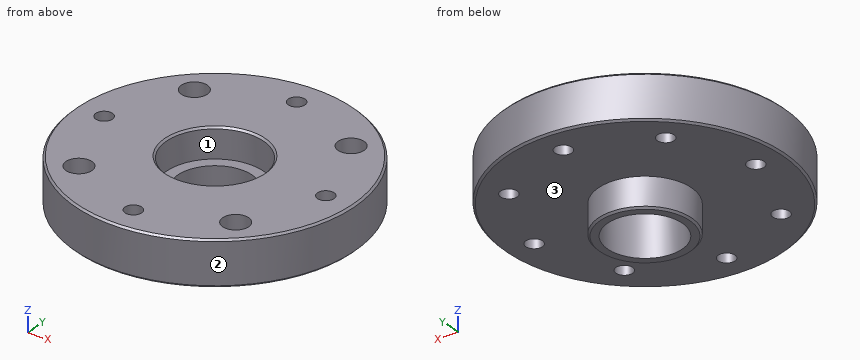
Solid Edge part; units mm, degrees
sketch "Sketch1" plane through (60.3162, 60.3162, 0) normal (0, 0, 1) x (1, 0, 0)
  circle A0 centre (-60.3162, -60.3162) radius 37.5
  circle A1 centre (-60.3162, -60.3162) radius 10
extrude "Protrusion1" add sketch "Sketch1" along normal blind 12
sketch "Sketch2" plane through (0, 0, 0) normal (0, 0, -1) x (1, 0, 0)
  circle A0 centre (0, 0) radius 10
  circle A1 centre (0, 0) radius 12.5
extrude "Extrusionsausprägung_2" add sketch "Sketch2" along normal blind 8
chamfer "Fase_1" distance 0.5 angle 45 1 edges at (-12.5, 0, -8)
hole "Bohrung_1" at (-30, 0, 12) direction (0, 0, -1) diameter 4.5 end through all
pattern_circular "Pattern1" count 8 over 360 about axis through (0, 0, 12) along (0, 0, 1) of "Bohrung_1"
chamfer "Fase_2" distance 0.5 angle 45 2 edges at (-37.5, 0, 12) (-37.5, 0, 0)
sketch "Sketch3" plane through (0, 0, 12) normal (0, 0, 1) x (-1, 0, 0)
  circle A0 centre (0, 0) radius 11
extrude "Extrusionsausprägung_4" add sketch "Sketch3" against normal blind 7
sketch "Sketch4" plane through (0, 0, 12) normal (0, 0, 1) x (-1, 0, 0)
  circle A0 centre (0, 0) radius 13
extrude "Extrusionsausschnitt_2" cut sketch "Sketch4" against normal blind 8
chamfer "Fase_3" distance 0.5 angle 45 1 edges at (13, 0, 12)
hole "Bohrung_2" at (-21.2132, -21.2132, 12) direction (0, 0, -1) diameter 4.5 end up to next counterbore diameter 7 counterbore depth 4
pattern_circular "Pattern3" count 4 over 360 about axis through (0, 0, 12) along (0, 0, -1) of "Bohrung_2"
properties material "Aluminium, 1060"
Design review of the part built by this model. Coordinates are the model's own, in mm. Face numbers are marked on the shaded views. A direction names the side the tool comes from. Round coordinates to 2 decimals unless told otherwise and drop trailing zeros. Order: outer loops, then holes, each group sorted by start corner. A loop starts at its lowest first (then second) coordinate and runs counter-clockwise, first axis right, second up. Notation, with made-up numbers: (56, 59.25) - (72, 59.25) arc R12 ccw to (72, 73.25) - close; hole circle Ø10 at (7, 36.5). An arc over 180 degrees is marked (long way). Return JSON: item names as keys, results as strings.
Q1. Consider section D-D on z = -5.75. Write out the cut boundary in (x, y).
Computed values:
{"outline": "circle Ø25 at (0, 0); hole circle Ø20 at (0, 0)"}
Q2. Wall thickness on L1, parallel to Y at x = 0, z = -1.75; L2, parallel to Z at x = -23.5, y = 15.5; L3, parallel to X at y = -3, z = -0.5: over which ranges is each line inside the solid? List them lowest first. Write a range as [from, to].
Computed values:
{"L1": "y = [-12.5, -10], [10, 12.5]", "L2": "z = [0, 12]", "L3": "x = [-12.13, -9.54], [9.54, 12.13]"}
Q3. Consider section A-A on x = 0. Give the number of separate pieces and of enclosed holes in the cut face, plus the area to 3 significant figures.
Computed values:
{"separate pieces": "4", "enclosed holes": "0", "area": "543 mm2"}
Q4. Machinability: for the marked faces 1, 2 and 3, which of the approach directions +Z, -Z, +X, -X, +Y, -Y give a long, thin tool a straight path to every point of the face, cutting with its end or side? Answer none if there is none.
Computed values:
{"face 1": "+Z", "face 2": "+Z, -Z", "face 3": "-Z"}
Q5. For pin 1 Ø13 at (x, y) = (5, 6.5) entering from +Z; pin 2 Ø11 at (x, y) = (21.21, -21.21) entering from -Z; pin 3 Ø5 at (y, z) = (-25.5, 4) entering from +X; pin 4 Ø8 at (y, z) = (-21.5, 0.5) entering from -X, all flat-tipped, find the tip position at first contact; note any pin that passes through.
Computed values:
{"pin 1": "stops at z = 12", "pin 2": "stops at z = 0", "pin 3": "stops at x = 29.62", "pin 4": "stops at x = -33.17"}
